Source: CAD feature listing. Evaluate the final solid. Frame: model axes, mm. Face numbers are marked on the shaded views. Coordinates: 2 decimals unless noted, no trailing zeros. Loops run counter-clockwise (first coordinate to the right, second up) from the corner with the lowest first, then second, coordinate; pieces in that order, holes last.
Item 1: Pin query (flat end, axial travel): pin 1 Ø3 at (x, z) = (52.5, -4.5) entering from -Y; pin 2 Ø5 at (x, y) = (33, 14.5) entering from -Z; pin 3 Ø5 at (y, z) = (16.5, -8) entering from +X. Return the tip coordinate at first contact, or that it passes through.
Item 2: Section query C-C, the plane x = 52. Return the cut outline in (y, z).
Item 3: Section query A-A, the plane y = 14. State how many separate pieces and enclosed holes the cut face has, then the cut area to 3 significant figures.
Item 4: Section query B-B, the plane z = -6.25. Return the cut outline in (x, y), then the cut area to 3 significant figures.
Item 5: Pull-direction query (X, two-part tool) for the marked faces 1 and 2; classes: +X half, -X half, draft (parallel to the pull), parting line (faces both ways), or undercut.
Item 6: Line query: probe 1 along X at (y, z) = (17, -9.5); probe 2 along X at (y, z) = (21.5, -2); probe 3 along Z at (x, y) = (24.5, 13.5). Output: solid intervals per line, ascending.
```python
from build123d import *

# Parameters (mm, degrees)
F0_W       = 105
F0_H       = 16.5
F1_DEPTH   = 2.5
F2_R       = 3.5
F2_R_2     = 1
F1_FACE1_W = 105
F1_FACE1_H = 16.5
F3_DEPTH   = 2.5
F5_R       = 4.5
F5_R_2     = 3.5
F6_DEPTH   = 9
F7_DEPTH   = 9


with BuildPart() as f1:
    # F0 (on Top) → F1 (new body)
    with BuildSketch(Plane.XY):
        with Locations((12.898709625, 16.1374760096)):
            Rectangle(F0_W, F0_H)
    extrude(amount=-F1_DEPTH)

    # F2 (on face) + F1_face1 (on face) → F3 (cut)
    with BuildSketch(Plane.XY):
        with BuildLine():
            ThreePointArc((33.4492198822, 24.3874760096), (34.5428361242, 18.6607738154), (39.398709625, 21.8874760096))
            ThreePointArc((39.398709625, 21.8874760096), (39.1254118192, 23.2433495104), (38.3481993678, 24.3874760096))
            Line((38.3481993678, 24.3874760096), (33.4492198822, 24.3874760096))
        make_face()
        with Locations((-4.6013260893, 16.0874760096)):
            Circle(F2_R)
        with Locations((14.3986739107, 16.0874760096)):
            Circle(F2_R)
        with Locations((-33.6013682725, 16.1680499117)):
            Circle(F2_R_2)
        with Locations((58.4004792942, 15.9800840236)):
            Circle(F2_R_2)
    with BuildSketch(Plane(origin=(12.898709625, 16.1374760096, -2.5), x_dir=(1, 0, 0), z_dir=(0, 0, -1))):
        Rectangle(F1_FACE1_W, F1_FACE1_H)
    extrude(amount=-F3_DEPTH, dir=(0, 0, 1), mode=Mode.SUBTRACT)

    # F5 (on face) → F6 (join)
    with BuildSketch(Plane(origin=(0, 0, -2.5), x_dir=(1, 0, 0), z_dir=(0, 0, -1))):
        with Locations((-4.5977425762, -16.0039048642)):
            Circle(F5_R)
        with Locations((-4.5977425762, -16.0039048642)):
            Circle(F5_R_2, mode=Mode.SUBTRACT)
        with Locations((14.3961599097, -16.0959586501)):
            Circle(F5_R)
        with Locations((14.3961599097, -16.0959586501)):
            Circle(F5_R_2, mode=Mode.SUBTRACT)
    extrude(amount=F6_DEPTH)

    # F5 (on face) → F7 (join)
    with BuildSketch(Plane(origin=(0, 0, -2.5), x_dir=(1, 0, 0), z_dir=(0, 0, -1))):
        with Locations((-4.5977425762, -16.0039048642)):
            Circle(F5_R)
        with Locations((-4.5977425762, -16.0039048642)):
            Circle(F5_R_2, mode=Mode.SUBTRACT)
        with Locations((14.3961599097, -16.0959586501)):
            Circle(F5_R)
        with Locations((14.3961599097, -16.0959586501)):
            Circle(F5_R_2, mode=Mode.SUBTRACT)
    extrude(amount=F7_DEPTH)


solid = f1.part
```
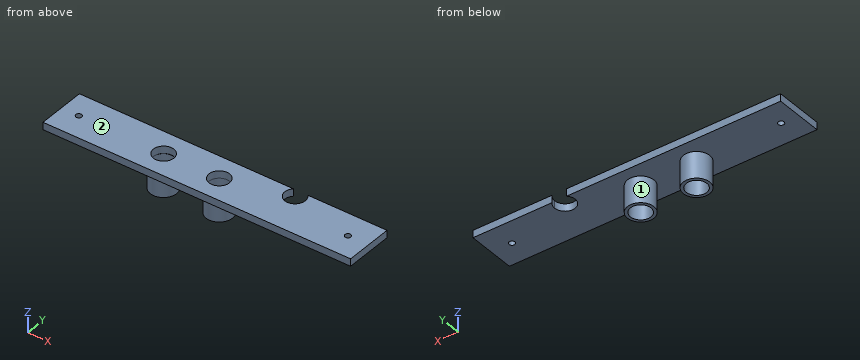
Verdict:
1. pin 1: passes through
1. pin 2: stops at z = -2.5
1. pin 3: stops at x = 18.9
2. outline: (7.89, -2.5) - (24.39, -2.5) - (24.39, 0) - (7.89, 0) - close
3. separate pieces: 3
3. enclosed holes: 0
3. area: 277 mm2
4. outline: circle Ø9 at (-4.6, 16); circle Ø9 at (14.4, 16.1); hole circle Ø7 at (-4.6, 16); hole circle Ø7 at (14.4, 16.1)
4. area: 50.3 mm2
5. face 1: undercut
5. face 2: draft
6. probe 1: x = -8.99 to -7.95, -1.24 to -0.21, 9.99 to 11.01, 17.78 to 18.8
6. probe 2: x = -39.6 to 32.42, 39.38 to 65.4
6. probe 3: z = -2.5 to 0
